The listing builds one solid part. Answer for the finished solid, in the listing's coordinates (mm). A direction names the side the tool comes from. Coordinates: 2 decimals unless noted, no trailing zeros. Write each loop counter-clockwise with the first axis right and the second up, starting at its lowest first coordinate (ties: lowest second). Pieces come first, ordered by that corner, then holes.
from build123d import *

# Parameters (mm, degrees)
SKETCH1_R           = 7.635
BOSS_EXTRUDE1_DEPTH = 26.95
BOSS_EXTRUDE1_DRAFT = -2
SKETCH5_W           = 30
SKETCH5_H           = 9
BOSS_EXTRUDE3_DEPTH = 24.9
SKETCH6_R           = 7.135
CUT_EXTRUDE1_DEPTH  = 37
CUT_EXTRUDE1_DRAFT  = 2
SKETCH7_W           = 15.3
SKETCH7_H           = 11.7
SKETCH7_W_2         = 10.82308768
SKETCH7_H_2         = 11.2
CUT_EXTRUDE2_DEPTH  = 38
CUT_EXTRUDE3_DEPTH  = 32
SKETCH9_R           = 1.25
CUT_EXTRUDE4_DEPTH  = 32
SKETCH10_W          = 17.5
SKETCH10_H          = 9.25
CUT_EXTRUDE5_DEPTH  = 15
SKETCH3_R           = 11.551989241
CUT_EXTRUDE6_DEPTH  = 1


with BuildPart() as part:
    # Sketch1 → Boss-Extrude1 (with draft: the straight prism first)
    with BuildSketch(Plane(origin=(0, 0, 0), x_dir=(1, 0, 0), z_dir=(0, 1, 0))):
        Circle(SKETCH1_R)
    extrude(amount=BOSS_EXTRUDE1_DEPTH)
    # Boss-Extrude1: the draft: its side faces are tilted about the plane it starts from
    boss_extrude1_sides = [part.faces().sort_by_distance(p)[0] for p in [
        (-7.635, 13.475, 0),
    ]]
    draft(boss_extrude1_sides, Plane(origin=(0, 0, 0), x_dir=(1, 0, 0), z_dir=(0, 1, 0)), BOSS_EXTRUDE1_DRAFT)

    # Sketch5 → Boss-Extrude3 (add)
    with BuildSketch(Plane.XY.offset(7)):
        with Locations((0, 10.29)):
            Rectangle(SKETCH5_W, SKETCH5_H)
    extrude(amount=BOSS_EXTRUDE3_DEPTH)


with BuildPart() as cut_extrude1_tool:
    # Sketch6 → Cut-Extrude1 (with draft: the straight prism first)
    with BuildSketch(Plane.XZ):
        Circle(SKETCH6_R)
    extrude(amount=-CUT_EXTRUDE1_DEPTH)
    # Cut-Extrude1: the draft: its side faces are tilted about the plane it starts from
    cut_extrude1_sides = [cut_extrude1_tool.faces().sort_by_distance(p)[0] for p in [
        (-7.135, 18.5, 0),
    ]]
    draft(cut_extrude1_sides, Plane.XZ, CUT_EXTRUDE1_DRAFT)


with BuildPart() as part_1:
    add(part.part)

    # Cut-Extrude1: cut by cut_extrude1_tool
    add(cut_extrude1_tool.part, mode=Mode.SUBTRACT)

    # Sketch7 → Cut-Extrude2 (cut)
    with BuildSketch(Plane(origin=(0, 14.79, 0), x_dir=(1, 0, 0), z_dir=(0, 1, 0))):
        with Locations((0, -26.05)):
            Rectangle(SKETCH7_W, SKETCH7_H)
        with Locations((9.58845616, -12.6)):
            Rectangle(SKETCH7_W_2, SKETCH7_H_2)
        with Locations((-9.58845616, -12.6)):
            Rectangle(SKETCH7_W_2, SKETCH7_H_2)
    extrude(amount=-CUT_EXTRUDE2_DEPTH, mode=Mode.SUBTRACT)

    # Sketch8 → Cut-Extrude3 (cut)
    with BuildSketch(Plane.ZY.offset(15)):
        Polygon((31.9, 6.79), (25.9, 14.79), (31.9, 14.79), align=None)
    extrude(amount=-CUT_EXTRUDE3_DEPTH, mode=Mode.SUBTRACT)

    # Sketch9 → Cut-Extrude4 (cut)
    with BuildSketch(Plane.ZY.offset(15)):
        with Locations(Location((26.353732334, 10.29, 0), (0, 0, 270))):
            Circle(SKETCH9_R)
    extrude(amount=-CUT_EXTRUDE4_DEPTH, mode=Mode.SUBTRACT)

    # Sketch10 → Cut-Extrude5 (cut)
    with BuildSketch(Plane.XY.offset(7)):
        with Locations((0, 19.575)):
            Rectangle(SKETCH10_W, SKETCH10_H)
    extrude(amount=CUT_EXTRUDE5_DEPTH, mode=Mode.SUBTRACT)

    # Sketch3 → Cut-Extrude6 (cut)
    with BuildSketch(Plane(origin=(0, 26.95, 0), x_dir=(1, 0, 0), z_dir=(0, 1, 0))):
        Circle(SKETCH3_R)
    extrude(amount=-CUT_EXTRUDE6_DEPTH, mode=Mode.SUBTRACT)


solid = part_1.part
1. For a pull along X with two mould halves and no side action, classify faces 4 (the flat face through (-4.177, 10, 13)), 5 (the flat face through (6.8, 0, 2.8)), 6 (the flat face through (7.65, 9, 25)) as pulls with the +X half, pulls with the -X half, needs draft (parallel to the pull), parting line crosses it, or undercut.
Results found:
face 4: pulls with the -X half
face 5: needs draft
face 6: undercut
2. Section C-C on x = 0 is taken. Give the vertices of the cut face in (y, z) (3 decimals).
Results found:
outline: (0, -7.635) - (25.95, -8.541) - (25.95, -8.041) - (0, -7.135) - close; (0, 7.135) - (14.95, 7.657) - (14.95, 8.157) - (14.79, 8.151) - (14.79, 20.2) - (5.79, 20.2) - (5.79, 7.837) - (0, 7.635) - close; (24.2, 7.98) - (25.95, 8.041) - (25.95, 8.541) - (24.2, 8.48) - close
3. Section D-D on z = 0 is taken. Give the vertices of the cut face in (x, y) (3 decimals).
Results found:
outline: (-8.541, 25.95) - (-7.635, 0) - (-7.135, 0) - (-8.041, 25.95) - close; (7.135, 0) - (7.635, 0) - (8.541, 25.95) - (8.041, 25.95) - close
4. Flat-ended cylindrical pins translate along their axes: P1, Ø10, axis at y = 11, z = 14, coming from the +X side; P2, Ø5, axis at y = 21.5, z = 6.5, coming from the +X side; P3, Ø4.5, axis at x = -3, y = 9.5, coming from the +Z side; P4, Ø12, axis at x = -7, z = 13.5, coming from the +Y side. Find the tip coordinate at first contact, or state that the pin passes through.
Results found:
P1: stops at x = 15
P2: stops at x = 7.37
P3: stops at z = 20.2
P4: stops at y = 14.79
5. Section A-A on y = 10.29 is taken. Give the vertices of the cut face in (x, z) (3 decimals), then the cut area to 3 significant figures.
Results found:
outline: (-15, 18.2) - (-4.177, 18.2) - (-4.177, 7) - (-3.861, 7) arc R7.994 ccw (long way) to (3.861, 7) - (4.177, 7) - (4.177, 18.2) - (15, 18.2) - (15, 25.104) - (7.65, 25.104) - (7.65, 20.2) - (-7.65, 20.2) - (-7.65, 25.104) - (-15, 25.104) - close; (-15, 27.604) - (-7.65, 27.604) - (-7.65, 29.275) - (-15, 29.275) - close; (7.65, 27.604) - (15, 27.604) - (15, 29.275) - (7.65, 29.275) - close; hole circle Ø14.989 at (0, 0)
area: 269 mm2
6. A tool of negligible diameter and unlimited length cuts with its end or side. For faces 1 (the flat face through (10, 10, 18.2)), 2 (the flat face through (4, 20, 7)), 3 (the conical face through (-1.644, 12.793, -7.401)), from which of +Z, -Z, +X, -X, +Y, -Y can it reach the whole face along a straight path? Write none if from no direction.
Results found:
face 1: +X, +Y, -Y
face 2: +Z, +X, -X
face 3: +Y
7. Find the intervals of material crossed by L1, parallel to Z at x = -6.5, y = 10.75; L2, parallel to X at y = 9, z = 29; L3, parallel to X at y = 16.25, z = 4.5, in increasing order.
Results found:
L1: z = -4.68 to -3.76, 3.76 to 4.68, 18.2 to 20.2
L2: x = -15 to -7.65, 7.65 to 15
L3: x = -6.86 to -6.25, 6.25 to 6.86
8. Section B-B on z = 27 is taken. Give the vertices of the cut face in (x, y).
Results found:
outline: (-15, 5.79) - (-7.65, 5.79) - (-7.65, 9.22) - (-15, 9.22) - close; (-15, 11.36) - (-7.65, 11.36) - (-7.65, 13.32) - (-15, 13.32) - close; (7.65, 5.79) - (15, 5.79) - (15, 9.22) - (7.65, 9.22) - close; (7.65, 11.36) - (15, 11.36) - (15, 13.32) - (7.65, 13.32) - close
